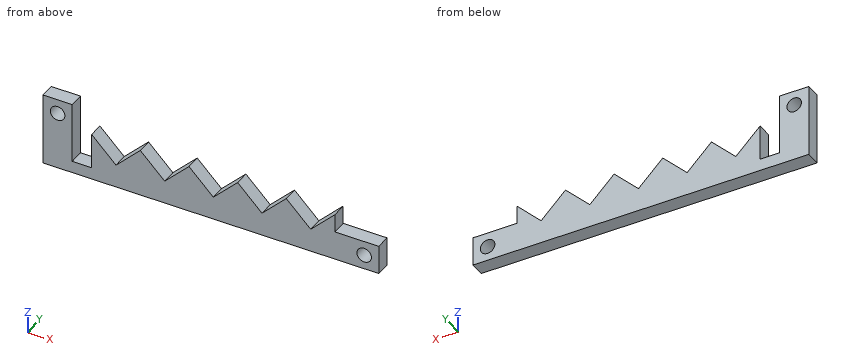
from build123d import *

# Parameters (mm, degrees)
SKETCH1_R           = 1.5
BOSS_EXTRUDE1_DEPTH = 3


with BuildPart() as part:
    # Sketch1 → Boss-Extrude1 (new body)
    with BuildSketch(Plane(origin=(0, 0, 0), x_dir=(1, 0, 0), z_dir=(0, 1, 0))):
        Polygon((0, 42.341154582), (0, 38.341154582), (5, 43.341154582), (10, 38.341154582), (15, 43.341154582), (20, 38.341154582), (25, 43.341154582), (30, 38.341154582), (35, 43.341154582), (40, 38.341154582), (45, 43.341154582), (50, 38.341154582), (50, 42.168762746), (59, 42.168762746), (59, 48.168762746), (58.943690308, 48.168762746), (5, 48.168762746), (-1.848815236, 48.168762746), (-10, 48.168762746), (-10, 33.168762746), (-4, 33.168762746), (-4, 45.696811654), (0, 45.696811654), align=None)
        with Locations((-7, 36.168762746)):
            Circle(SKETCH1_R, mode=Mode.SUBTRACT)
        with Locations((56, 45.168762746)):
            Circle(SKETCH1_R, mode=Mode.SUBTRACT)
    extrude(amount=BOSS_EXTRUDE1_DEPTH)


solid = part.part
Source: CAD feature listing. Evaluate the final solid. Frame: model axes, mm. Round coordinates to 2 decimals unless told otherwise and drop trailing zeros. Write each loop counter-clockwise with the first axis right and the second up, starting at its lowest first coordinate (ties: lowest second). Pieces come first, ordered by that corner, then holes. Notation, with made-up numbers: (74.5, 39.25) - (96.5, 39.25) arc R27 cw to (96.5, 67.25) - close; hole circle Ø9 at (85.5, -39). An arc over 180 degrees is marked (long way). Use CSV: the item, a comma, the result in double quotes. Start each with the question number.
(1) First-contact query: pin 1 Ø6 at (x, z) = (25.5, -36.5) entering from -Y; pin 2 Ø1.5 at (x, y) = (48.5, 2.5) entering from +Z. Flat tips, straight axial feed; report the tip coordinate or a pass-through.
(2) Cut plane C-C, the plane y = 2.5. Return loops of the section in (x, z), and give its area (3 significant figures).
(3) Cut plane A-A, the plane x = 56. Return loops of the section in (y, z).
(4) Cut plane D-D, the plane z = -33.75. Return loops of the section in (x, y).
(5) Material intervals for probe 1 along Z at (x, y) = (-7, 1.7); probe 2 along X at (y, z) = (2.3, -36.5); probe 3 along X at (y, z) = (0.9, -35.75), sorted ascending. Write a range as [from, to].
(6) Cut plane B-B, the plane x = -7. Return loops of the section in (y, z), and give its area (3 significant figures).
Geometry says:
1,pin 1,"through"
1,pin 2,"z = -39.09"
2,outline,"(-10, -48.17) - (59, -48.17) - (59, -42.17) - (50, -42.17) - (50, -38.34) - (45, -43.34) - (40, -38.34) - (35, -43.34) - (30, -38.34) - (25, -43.34) - (20, -38.34) - (15, -43.34) - (10, -38.34) - (5, -43.34) - (0, -38.34) - (0, -45.7) - (-4, -45.7) - (-4, -33.17) - (-10, -33.17) - close; hole circle Ø3 at (-7, -36.17); hole circle Ø3 at (56, -45.17)"
2,area,"506 mm²"
3,outline,"(0, -48.17) - (3, -48.17) - (3, -46.67) - (0, -46.67) - close; (0, -43.67) - (3, -43.67) - (3, -42.17) - (0, -42.17) - close"
4,outline,"(-10, 0) - (-4, 0) - (-4, 3) - (-10, 3) - close"
5,probe 1,"[-48.17, -37.67], [-34.67, -33.17]"
5,probe 2,"[-10, -8.46], [-5.54, -4]"
5,probe 3,"[-10, -8.44], [-5.56, -4]"
6,outline,"(0, -48.17) - (3, -48.17) - (3, -37.67) - (0, -37.67) - close; (0, -34.67) - (3, -34.67) - (3, -33.17) - (0, -33.17) - close"
6,area,"36.0 mm²"
